Could you check a few things on this model? Use its own coordinates, in mm. A direction names the side the tool comes from. Round coordinates to 2 decimals unless told otherwise and drop trailing zeros. Loops run counter-clockwise (first coordinate to the right, second up) from the corner with the lowest first, then second, coordinate; pieces in that order, holes last. Notation, with made-up numbers: (66, 55) -> (80, 55) arc R22 cw to (80, 64) -> close; hole circle Ø11 at (74.25, -21.5). An arc over 180 degrees is marked (long way). Write each question's results on one line, items separated by ' | '. Start each with the question number.
1) Imagine slicing it at C-C, the plane z = 0.5. List the corners of the cut face in (x, y) for me.
2) Imagine slicing it at B-B, the plane z = -2.5. List the corners of the cut face in (x, y) for me.
3) Which directions (+Z, -Z, +X, -X, +Y, -Y) give clear straight access to the entire face, cutting with the end or side of a thin tool? Please do faces 1 (the cylindrical face through (4.5, 4.1, 0.6)), 2 (the flat face through (15, 5, -2)), 3 (the flat face through (6, 5, 3)).
4) We'd pull the mould along X, two halves only. Please class faces 4 (the cylindrical face through (3.9, -4.7, 3.5)), 5 (the flat face through (15.7, 7.5, 0.5)), 6 (the cylindrical face through (26.5, -0.16, 0.49)), 7 (the cylindrical face through (11.5, 7.2, 0.8)): pulls with the +X half, pulls with the -X half, needs draft (parallel to the pull), parting line crosses it, or undercut.
5) For P1, Ø2.5, axis at x = 7.5, z = 3.5, coming from the -Y side; P2, Ø3, axis at y = -3.5, z = -2.5, coming from the +X side; P3, Ø0.6, axis at x = 12.5, z = 2, coming from the -Y side; P4, Ø0.6, axis at y = 5.5, z = 2.5, coming from the -X side, each with a flat end and sliding along its axis, tell me the tip position at first contact or that it passes through.
6) If I drill on probe 1 along X at (y, z) = (0, -0.5); probe 2 along X at (y, z) = (-2, 3.5); probe 3 along Y at (x, z) = (20.5, 1.5), over which ranges is the centre line in solid material (lowest first)?
7) Imagine slicing it at A-A, the plane y = 0. List the corners of the cut face in (x, z) for me, plus the area to 3 significant figures.
from build123d import *

# Parameters (mm, degrees)
F0_W     = 22.6132244859
F0_H     = 0.6
F0_W_2   = 4.1867755141
F0_W_3   = 10
F0_W_4   = 3
F1_DEPTH = 2
F2_DEPTH = 4
F3_START = -3
F3_DEPTH = 1
F4_DEPTH = 5
F5_R     = 1


with BuildPart() as f1:
    # F0 (on Top) → F1 (new body)
    with BuildSketch(Plane.XY):
        with BuildLine():
            ThreePointArc((-19, -5.6), (-24.6, 0), (-19, 5.6))
            Line((-19, 5.6), (3.6132244859, 5.6))
            Line((3.6132244859, 5.6), (7.2132244859, 5.6))
            Line((7.2132244859, 5.6), (7.2132244859, 7.5))
            Line((7.2132244859, 7.5), (-19, 7.5))
            ThreePointArc((-19, 7.5), (-26.5, 0), (-19, -7.5))
            Line((-19, -7.5), (19, -7.5))
            ThreePointArc((19, -7.5), (26.5, 0), (19, 7.5))
            Line((19, 7.5), (11.2132244859, 7.5))
            Line((11.2132244859, 7.5), (11.2132244859, 5.6))
            Line((11.2132244859, 5.6), (14.8132244859, 5.6))
            Line((14.8132244859, 5.6), (19, 5.6))
            ThreePointArc((19, 5.6), (24.6, 0), (19, -5.6))
            Line((19, -5.6), (14.8132244859, -5.6))
            Line((14.8132244859, -5.6), (3.6132244859, -5.6))
            Line((3.6132244859, -5.6), (-19, -5.6))
        make_face()
        with Locations((-7.6933877571, 5.3)):
            Rectangle(F0_W, F0_H)
        with Locations((16.9066122429, 5.3)):
            Rectangle(F0_W_2, F0_H)
        with Locations((-7.6933877571, -5.3)):
            Rectangle(F0_W, F0_H)
        with Locations((16.9066122429, -5.3)):
            Rectangle(F0_W_2, F0_H)
        with BuildLine():
            Line((3.6132244859, 5), (-19, 5))
            ThreePointArc((-19, 5), (-24, 0), (-19, -5))
            Line((-19, -5), (3.6132244859, -5))
            Line((3.6132244859, -5), (3.6132244859, 5))
        make_face()
        Polygon((4.2132244859, 5), (3.6132244859, 5), (3.6132244859, -5), (4.2132244859, -5), (4.2132244859, -4.4), (4.2132244859, 4.4), align=None)
        Polygon((3.6132244859, 5.6), (3.6132244859, 5), (4.2132244859, 5), (7.2132244859, 5), (7.2132244859, 5.6), align=None)
        with BuildLine():
            Line((14.8132244859, 5), (14.8132244859, -5))
            Line((14.8132244859, -5), (19, -5))
            ThreePointArc((19, -5), (24, 0), (19, 5))
            Line((19, 5), (14.8132244859, 5))
        make_face()
        Polygon((4.2132244859, -5), (3.6132244859, -5), (3.6132244859, -5.6), (14.8132244859, -5.6), (14.8132244859, -5), (14.2132244859, -5), align=None)
        Polygon((14.2132244859, -4.4), (14.2132244859, -5), (14.8132244859, -5), (14.8132244859, 5), (14.2132244859, 5), (14.2132244859, 4.4), align=None)
        Polygon((14.2132244859, 5), (14.8132244859, 5), (14.8132244859, 5.6), (11.2132244859, 5.6), (11.2132244859, 5), align=None)
        with Locations((9.2132244859, -4.7)):
            Rectangle(F0_W_3, F0_H)
        with Locations((5.7132244859, 4.7)):
            Rectangle(F0_W_4, F0_H)
        with Locations((12.7132244859, 4.7)):
            Rectangle(F0_W_4, F0_H)
    extrude(amount=F1_DEPTH)

    # F0 (on Top) → F2 (join)
    with BuildSketch(Plane.XY):
        with BuildLine():
            Line((3.6132244859, 5), (-19, 5))
            ThreePointArc((-19, 5), (-24, 0), (-19, -5))
            Line((-19, -5), (3.6132244859, -5))
            Line((3.6132244859, -5), (3.6132244859, 5))
        make_face()
        with BuildLine():
            Line((14.8132244859, 5), (14.8132244859, -5))
            Line((14.8132244859, -5), (19, -5))
            ThreePointArc((19, -5), (24, 0), (19, 5))
            Line((19, 5), (14.8132244859, 5))
        make_face()
        Polygon((4.2132244859, 5), (3.6132244859, 5), (3.6132244859, -5), (4.2132244859, -5), (4.2132244859, -4.4), (4.2132244859, 4.4), align=None)
        Polygon((14.2132244859, -4.4), (14.2132244859, -5), (14.8132244859, -5), (14.8132244859, 5), (14.2132244859, 5), (14.2132244859, 4.4), align=None)
        with Locations((9.2132244859, -4.7)):
            Rectangle(F0_W_3, F0_H)
        with Locations((5.7132244859, 4.7)):
            Rectangle(F0_W_4, F0_H)
        with Locations((12.7132244859, 4.7)):
            Rectangle(F0_W_4, F0_H)
    extrude(amount=-F2_DEPTH)

    # F0 (on Top) → F3 (join)
    with BuildSketch(Plane.XY.offset(F3_START)):
        with BuildLine():
            ThreePointArc((-19, -5), (-24, 0), (-19, 5))
            Line((-19, 5), (-19, 5.6))
            ThreePointArc((-19, 5.6), (-24.6, 0), (-19, -5.6))
            Line((-19, -5.6), (-19, -5))
        make_face()
        with BuildLine():
            Line((19, -5), (19, -5.6))
            ThreePointArc((19, -5.6), (24.6, 0), (19, 5.6))
            Line((19, 5.6), (19, 5))
            ThreePointArc((19, 5), (24, 0), (19, -5))
        make_face()
    extrude(amount=-F3_DEPTH)

    # F0 (on Top) → F4 (join)
    with BuildSketch(Plane.XY):
        Polygon((4.2132244859, 5), (3.6132244859, 5), (3.6132244859, -5), (4.2132244859, -5), (4.2132244859, -4.4), (4.2132244859, 4.4), align=None)
        Polygon((14.2132244859, -4.4), (14.2132244859, -5), (14.8132244859, -5), (14.8132244859, 5), (14.2132244859, 5), (14.2132244859, 4.4), align=None)
        with Locations((9.2132244859, -4.7)):
            Rectangle(F0_W_3, F0_H)
        with Locations((5.7132244859, 4.7)):
            Rectangle(F0_W_4, F0_H)
        with Locations((12.7132244859, 4.7)):
            Rectangle(F0_W_4, F0_H)
    extrude(amount=F4_DEPTH)

    # F5
    f5_edges = [f1.edges().sort_by_distance(p)[0] for p in [
        (11.213224, 7.5, 1),
        (7.213224, 7.5, 1),
        (0, -7.5, 2),
        (4.213224, -4.4, 0.5),
        (14.213224, -4.4, 0.5),
        (3.613224, -5, 3.5),
        (14.813224, -5, 3.5),
        (14.813224, 5, 3.5),
        (3.613224, 5, 3.5),
        (4.213224, 4.4, 0.5),
        (14.213224, 4.4, 0.5),
    ]]
    fillet(f5_edges, radius=F5_R)


solid = f1.part
Checked values:
1) outline: (-19, -7.5) -> (19, -7.5) arc R7.5 ccw to (19, 7.5) -> (12.21, 7.5) arc R1 ccw to (11.21, 6.5) -> (11.21, 4.4) -> (13.21, 4.4) arc R1 cw to (14.21, 3.4) -> (14.21, -3.4) arc R1 cw to (13.21, -4.4) -> (5.21, -4.4) arc R1 cw to (4.21, -3.4) -> (4.21, 3.4) arc R1 cw to (5.21, 4.4) -> (7.21, 4.4) -> (7.21, 6.5) arc R1 ccw to (6.21, 7.5) -> (-19, 7.5) arc R7.5 ccw to start; hole (-19, -5.6) -> (-19, -5) arc R5 cw to (-19, 5) -> (-19, 5.6) arc R5.6 ccw to start; hole (19, -5.6) arc R5.6 ccw to (19, 5.6) -> (19, 5) arc R5 cw to (19, -5) -> close
2) outline: (-19, -5) -> (19, -5) arc R5 ccw to (19, 5) -> (11.21, 5) -> (11.21, 4.4) -> (13.21, 4.4) arc R1 cw to (14.21, 3.4) -> (14.21, -3.4) arc R1 cw to (13.21, -4.4) -> (5.21, -4.4) arc R1 cw to (4.21, -3.4) -> (4.21, 3.4) arc R1 cw to (5.21, 4.4) -> (7.21, 4.4) -> (7.21, 5) -> (-19, 5) arc R5 ccw to start
3) face 1: +Z, -Z | face 2: -Z, +Y | face 3: +Z, +X, -X, +Y
4) face 4: pulls with the -X half | face 5: needs draft | face 6: pulls with the +X half | face 7: undercut
5) P1: y = -5 | P2: x = 24.2 | P3: y = -7.21 | P4: through
6) probe 1: -24 to 4.21, 14.21 to 24 | probe 2: 3.61 to 4.21, 14.21 to 14.81 | probe 3: -7.21 to -5.4, -4.77 to 4.77, 5.4 to 7.21
7) outline: (-26.5, 0) -> (-24.6, 0) -> (-24.6, 2) -> (-25.5, 2) arc R1 ccw to (-26.5, 1) -> close; (-24.6, -4) -> (4.21, -4) -> (4.21, 5) -> (3.61, 5) -> (3.61, 2) -> (-24, 2) -> (-24, -3) -> (-24.6, -3) -> close; (14.21, -4) -> (24.6, -4) -> (24.6, -3) -> (24, -3) -> (24, 2) -> (14.81, 2) -> (14.81, 5) -> (14.21, 5) -> close; (24.6, 0) -> (26.5, 0) -> (26.5, 1) arc R1 ccw to (25.5, 2) -> (24.6, 2) -> close | area: 240 mm^2
